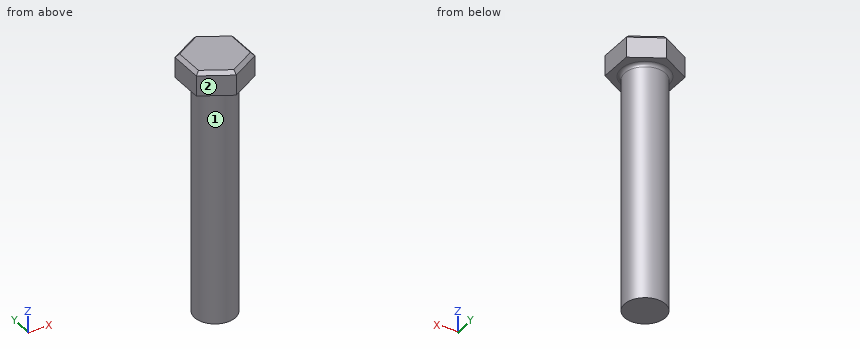
from build123d import *

# Parameters (mm, degrees)
CROQUIS1_R              = 6
SALIENTE_EXTRUIR3_DEPTH = 70
SALIENTE_EXTRUIR4_DEPTH = 7
CHAFL_N1_SIZE           = 1
REDONDEO1_R             = 1


with BuildPart() as part:
    # Croquis1 → Saliente-Extruir3 (new body)
    with BuildSketch(Plane.XY):
        Circle(CROQUIS1_R)
    extrude(amount=SALIENTE_EXTRUIR3_DEPTH)

    # Croquis3 → Saliente-Extruir4 (add)
    with BuildSketch(Plane.XY.offset(70)):
        Polygon((0, 10), (-8.660254038, 5), (-8.660254038, -5), (0, -10), (8.660254038, -5), (8.660254038, 5), align=None)
    extrude(amount=SALIENTE_EXTRUIR4_DEPTH)

    # Chaflán1
    chafl_n1_edges = [part.edges().sort_by_distance(p)[0] for p in [
        (8.660254038, 0, 77),
        (4.330127019, 7.5, 77),
        (-4.330127019, 7.5, 77),
        (-8.660254038, 0, 77),
        (-4.330127019, -7.5, 77),
        (4.330127019, -7.5, 77),
    ]]
    chamfer(chafl_n1_edges, length=CHAFL_N1_SIZE)

    # Redondeo1
    redondeo1_edges = [part.edges().sort_by_distance(p)[0] for p in [
        (-6, 0, 70),
    ]]
    fillet(redondeo1_edges, radius=REDONDEO1_R)


solid = part.part
Design review of the part built by this model. Coordinates are the model's own, in mm. Face numbers are marked on the shaded views. A direction names the side the tool comes from. Round coordinates to 2 decimals unless told otherwise and drop trailing zeros. Write each loop counter-clockwise with the first axis right and the second up, starting at its lowest first coordinate (ties: lowest second). Pieces come first, ordered by that corner, then holes. Notation, with made-up numbers: (50, 55) -> (58, 55) arc R11 cw to (58, 70) -> close; hole circle Ø3 at (49.25, -24). An arc over 180 degrees is marked (long way). One line per item, written item: value. Start each with the question number.
Q1. Tool access review of the marked faces 1 and 2: name each direction out of +Z, -Z, +X, -X, +Y, -Y from which nothing blocks a thin tool from reaching the whole face with its end or side.
Q2. Insertion check: P1, Ø3, axis at y = -2.5, z = 12.5, coming from the -X side; P2, Ø6, axis at x = 4, z = 15.5, coming from the +Y side; P3, Ø12, axis at y = 4.5, z = 31, coming from the -X side. Each pin has a flat end and moves straight along its axis. Give the tip position at first contact, or say it passes through.
Q3. Add section B-B (z = 32). Give the boundary of the cut face in (x, y).
Q4. To check wall thickness, follow probe 1 along Z at (x, y) = (-5.75, -3.75); probe 2 along Y at (x, z) = (-1.75, 41); probe 3 along Z at (x, y) = (-7.75, 3.25). State the ranges of each line that lie inside material, in increasing order.
Q5. Add section A-A (y = 0). Give the boundary of the cut face in (x, z).
Response:
1. face 1: -Z
1. face 2: +Z, -Z, -X, -Y
2. P1: stops at x = -5.92
2. P2: stops at y = 5.92
2. P3: stops at x = -6
3. outline: circle Ø12 at (0, 0)
4. probe 1: z = 69.99 to 77
4. probe 2: y = -5.74 to 5.74
4. probe 3: z = 70 to 76.91
5. outline: (-8.66, 70) -> (-7, 70) arc R1 cw to (-6, 69) -> (-6, 0) -> (6, 0) -> (6, 69) arc R1 cw to (7, 70) -> (8.66, 70) -> (8.66, 76) -> (7.66, 77) -> (-7.66, 77) -> (-8.66, 76) -> close
